The drawing under review shows one solid part. Ordinate dimensions are in mm from its lowest x, y, z. A direction names the side the tool comes from. Coordinates: 2 decimals unless noted, no trailing zeros. Write each loop counter-clockwise with the first axis right and the second up, starting at its lowest first coordinate (ties: lowest second). Pieces come first, ordered by that corner, then holes.
Q1. The part is to be moulded in two halves that separate along Y. For the marked faces 1, 2 and 3, say which applies: +Y half, -Y half, draft (parallel to the pull), parting line (faces both ways), or undercut.
Q2. Add section A-A, the plane z = 9. Give the boundary of the cut face in (x, y).
Q3. To check wall thickness, follow probe 1 along X at (y, z) = (10, 6.5); probe 2 along Y at (x, z) = (19.5, 6); probe 3 along X at (y, z) = (24.5, 7). State the ranges of each line that lie inside material, in increasing order.
Q4. Add section C-C, the plane y = 23.5. Give the boundary of the cut face in (x, z).
Q5. Machinability: for the marked faces 4 and 5, which of the approach directions +Z, -Z, +X, -X, +Y, -Y give a long, thin tool a straight path to every point of the face, cutting with its end or side? Answer none if there is none.
Q6. Add section B-B, the plane x = 29.9. Give the boundary of the cut face in (y, z), plus the area to 3 significant figures.
Q7. Add section D-D, the plane x = 17. Give the boundary of the cut face in (y, z).
Q8. Clearance check with a flat-ended pin moving along its axis: pin 1 Ø4.5 at (x, z) = (16, 8.5) entering from -Y. State where the tip first meets the part, or that it passes through.
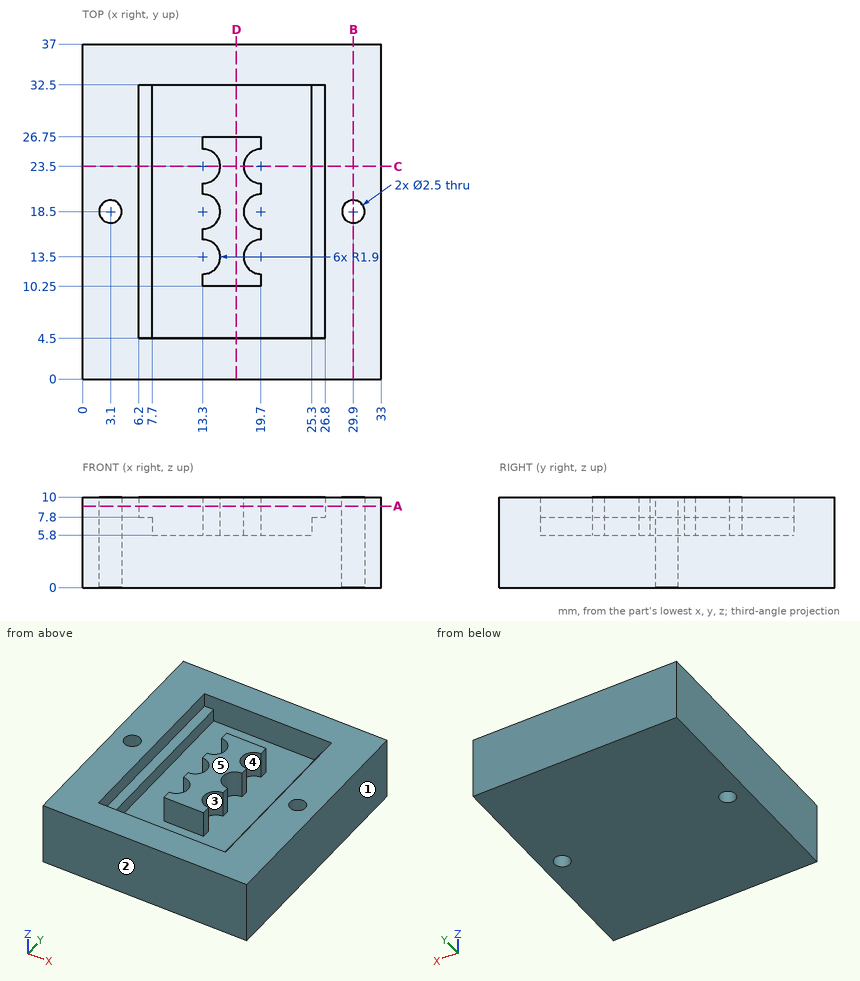
Here are the results:
1. face 1: draft
1. face 2: -Y half
1. face 3: undercut
2. outline: (0, 0) - (33, 0) - (33, 37) - (0, 37) - close; (13.3, 10.25) - (19.7, 10.25) - (19.7, 11.6) arc R1.9 cw to (19.7, 15.4) - (19.7, 16.6) arc R1.9 cw to (19.7, 20.4) - (19.7, 21.6) arc R1.9 cw to (19.7, 25.4) - (19.7, 26.75) - (13.3, 26.75) - (13.3, 25.4) arc R1.9 cw to (13.3, 21.6) - (13.3, 20.4) arc R1.9 cw to (13.3, 16.6) - (13.3, 15.4) arc R1.9 cw to (13.3, 11.6) - close; hole circle Ø2.5 at (3.1, 18.5); hole (6.2, 4.5) - (26.8, 4.5) - (26.8, 32.5) - (6.2, 32.5) - close; hole circle Ø2.5 at (29.9, 18.5)
3. probe 1: x = 0 to 7.7, 25.3 to 33
3. probe 2: y = 0 to 4.5, 10.25 to 11.61, 15.39 to 16.61, 20.39 to 21.61, 25.39 to 26.75, 32.5 to 37
3. probe 3: x = 0 to 7.7, 14.92 to 18.08, 25.3 to 33
4. outline: (0, 0) - (33, 0) - (33, 10) - (26.8, 10) - (26.8, 7.8) - (25.3, 7.8) - (25.3, 5.8) - (17.8, 5.8) - (17.8, 10) - (15.2, 10) - (15.2, 5.8) - (7.7, 5.8) - (7.7, 7.8) - (6.2, 7.8) - (6.2, 10) - (0, 10) - close
5. face 4: +Z
5. face 5: +Z, +X, -X, +Y, -Y
6. outline: (0, 0) - (17.25, 0) - (17.25, 10) - (0, 10) - close; (19.75, 0) - (37, 0) - (37, 10) - (19.75, 10) - close
6. area: 345 mm2
7. outline: (0, 0) - (37, 0) - (37, 10) - (32.5, 10) - (32.5, 5.8) - (26.75, 5.8) - (26.75, 10) - (10.25, 10) - (10.25, 5.8) - (4.5, 5.8) - (4.5, 10) - (0, 10) - close
8. pin 1: stops at y = 0
